Autodesk Inventor part; units mm, degrees
ref_plane "YZ Plane" through (0, 0, 0) normal (1, 0, 0) x (0, 1, 0)
ref_plane "XZ Plane" through (0, 0, 0) normal (0, 1, 0) x (-1, 0, 0)
ref_plane "XY Plane" through (0, 0, 0) normal (0, 0, 1) x (1, 0, 0)
sketch "Sketch1" plane through (0, 0, 0) normal (0, 1, 0) x (-1, 0, 0)
  arc A0 (4.6831, -2.7877) -> (-4.2282, 3.4387) centre (0, 0) ccw
  line L0 (4.6831, -2.7877) -> (-6.0873, -20.8805)
  line L1 (-4.2282, 3.4387) -> (-7.9464, -1.1331)
  arc A1 (-15.3196, -26.129) -> (-6.0873, -20.8805) centre (-15.3196, -15.3847) ccw
  arc A2 (-15.3196, -4.6405) -> (-7.9464, -1.1331) centre (-15.3196, 4.8633) ccw
  line L2 (-15.3196, -26.129) -> (-189.4823, -26.129)
  line L3 (-15.3196, -4.6405) -> (-189.4823, -4.6405)
  arc A3 (-194.5547, 0.2259) -> (-205.3394, -1.0922) centre (-200, 0) ccw
  arc A4 (-194.5547, 0.2259) -> (-189.4823, -4.6405) centre (-189.4823, 0.4363) ccw
  arc A5 (-202.3696, -15.6109) -> (-189.4823, -26.129) centre (-189.4823, -12.9748) ccw
  line L4 (-202.3696, -15.6109) -> (-205.3394, -1.0922)
  point P0 (-6.0873, 1.1528)
  point P1 (-10.0096, -24.7251)
  point P2 (-0.7021, -11.8341)
  dimension "d0" = 10.9
  dimension "d1" = 10.9
  dimension "d2" = 200
  dimension "d3" = 0
  dimension "d6" = 0
  dimension "d7" = 0
  dimension "d8" = 0
  dimension "d9" = 174.1627
  dimension "d10" = 9.3075
  dimension "d11" = 13.1542
extrude "Extrusion1" add sketch "Sketch1" along normal blind 1.7
sketch "Sketch2" plane through (0, 1.7, 0) normal (0, 1, 0) x (1, 0, 0)
  arc A0 (-4.6831, 2.7877) -> (4.2282, -3.4387) centre (0, 0) ccw
  circle A1 centre (0, 0) radius 1.5
  arc A2 (194.5547, -0.2259) -> (205.3394, 1.0922) centre (200, 0) ccw
  circle A3 centre (200, 0) radius 1.5
  dimension "d14" = 3
  dimension "d15" = 3
extrude "Extrusion2" cut sketch "Sketch2" against normal blind 1.7
equation "\"BendRadius\" = Thickness"
equation "\"BendReliefWidth\" = Thickness"
equation "\"BendReliefDepth\" = 0.5 * Thickness"
equation "\"CornerReliefSize\" = 4 * Thickness"
equation "\"MinimumRemnant\" = 2 * Thickness"
equation "\"TransitionRadius\" = BendRadius"
equation "\"JacobiRadiusSize\" = BendRadius"
equation "\"GapSize\" = Thickness"
properties part number "A3P1"
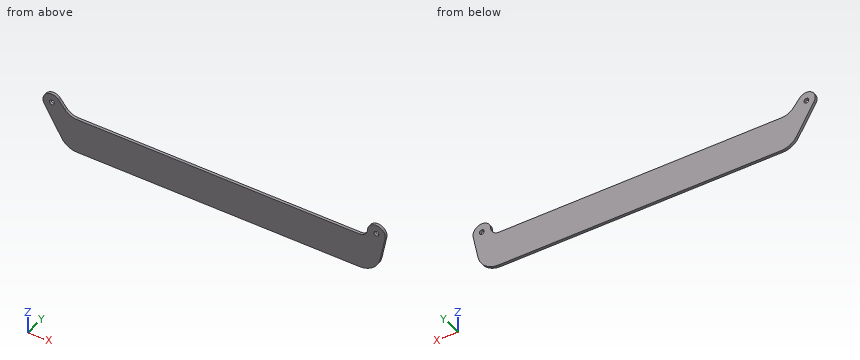
Work out the finished part from the listing and answer in its coordinate system (mm). Give positions to 0.01 mm unless a question says otherwise; leave off trailing zeros. Order: outer loops, then holes, each group sorted by start corner. A loop starts at its lowest first (then second) coordinate and runs counter-clockwise, first axis right, second up. Notation, with made-up numbers: (13.25, -34.5) - (20.25, -34.5) arc R36 ccw to (20.25, 4.5) - close; hole circle Ø4 at (25, 17.25). An arc over 180 degrees is marked (long way). One line per item, written item: value. Start each with the question number.
1. Section C-C, the plane z = -8 is taken. Write down the section's boundary in (x, y), then the cut area to 3 significant figures.
2. Section B-B, the plane x = 63 is taken. Write down the section's boundary in (y, z).
3. Section A-A, the plane y = 1.4 is taken. Write down the section's boundary in (x, z), then the cut area to 3 significant figures.
4. Each of these flat-tipped pins is pushed along its axis until it touches: pin 1 Ø2.5 at (x, z) = (200, 0) entering from +Y; pin 2 Ø0.8 at (x, y) = (122, 0.5) entering from +Z. Where does it stop, or does it pass through?
5. Consider line 1 (Z direction, x = 200, y = 0.9); line 2 (X direction, y = 1.2, z = 0); line 3 (Z direction, x = 91.5, y = 0.95). Determine where each line is inside the solid, lowest interval first.
Filled sheet:
1. outline: (-1.58, 0) - (203.93, 0) - (203.93, 1.7) - (-1.58, 1.7) - close
1. area: 349 mm²
2. outline: (0, -26.13) - (1.7, -26.13) - (1.7, -4.64) - (0, -4.64) - close
3. outline: (-4.68, -2.79) - (6.09, -20.88) arc R10.74 ccw to (15.32, -26.13) - (189.48, -26.13) arc R13.15 ccw to (202.37, -15.61) - (205.34, -1.09) arc R5.45 ccw (long way) to (194.55, 0.23) arc R5.08 cw to (189.48, -4.64) - (15.32, -4.64) arc R9.5 cw to (7.95, -1.13) - (4.23, 3.44) arc R5.45 ccw to start; hole circle Ø3 at (0, 0); hole circle Ø3 at (200, 0)
3. area: 4,460 mm²
4. pin 1: through
4. pin 2: z = -4.64
5. line 1: -20.87 to -1.5, 1.5 to 5.45
5. line 2: -5.45 to -1.5, 1.5 to 7.02, 194.54 to 198.5, 201.5 to 205.45
5. line 3: -26.13 to -4.64
